Input: part model. Units: mm. Frame: model coordinates. A direction names the side the tool comes from. Round coordinates to 2 decimals unless told otherwise and drop trailing zeros. Order: outer loops, then holes, each group sorted by start corner. A loop starts at its lowest first (then second) coordinate and runs counter-clockwise, first axis right, second up. Notation, with made-up numbers: (39.5, 55.5) -> (62.5, 55.5) arc R4 ccw to (62.5, 61.5) -> close; hole circle Ø6 at (-14.5, 27.25). An arc over 180 degrees is marked (long way). Answer as CSV lines item,"result". Start each with the question number.
1) Section query A-A, the plane z = 44. Output: boundary loops of the cut face in (x, y), and give its area (3 significant figures).
2) Section query C-C, the plane y = 9. Output: boundary loops of the cut face in (x, z).
3) First-contact query: P1, Ø22, axis at y = 5, z = 32.5, coming from the -X side; P2, Ø16, axis at x = 28.5, y = 13, coming from the +Z side; P3, Ø5, axis at x = 25.5, z = 7.5, coming from the +Y side; P4, Ø6, axis at x = 46, y = 29.5, coming from the -Z side. Flat tips, straight axial feed; report the tip coordinate or a pass-through.
4) Line query: L1, parallel to X at y = 26.5, z = -34; L2, parallel to Y at x = 18, z = 19; L3, parallel to Y at x = 41, z = -26.5. Output: solid intervals per line, ascending.
5) Section query D-D, the plane x = 62.5. Output: boundary loops of the cut face in (y, z), and give its area (3 significant figures).
6) Access query for faces 1 (the face through (15, 20, -45)), 2 (the face through (20, 32, -30)), 3 (the face through (62.605, 9.86, 24.65)), 4 (the face through (50, 10, 35)), 5 (the face through (35, 23, -20)). Directions: +Z, -Z, +X, -X, +Y, -Y. A direction counts if a zero-diameter tool reaches every point of the face in a straight line with its end or side. Return the directions, or none.
7) Section query B-B, the plane y = 28.5. Output: boundary loops of the cut face in (x, z), and give its area (3 significant figures).
```python
from build123d import *

# Parameters (mm, degrees)
BOSS_EXTRUDE1_DEPTH = 20
SKETCH2_W           = 70
SKETCH2_H           = 30
BOSS_EXTRUDE2_DEPTH = 20
CUT_EXTRUDE1_REACH  = 96.868
SKETCH3_W           = 40
SKETCH3_H           = 10
CUT_EXTRUDE2_REACH  = 108.771
SKETCH4_W           = 30
SKETCH4_H           = 15


with BuildPart() as part:
    # Sketch1 → Boss-Extrude1 (new body)
    with BuildSketch(Plane(origin=(0, 0, 0), x_dir=(1, 0, 0), z_dir=(0, 1, 0))):
        Polygon((0, 0), (0, 50), (70, 50), (70, 0), (55, -50), (50, -50), (50, -20), (20, -20), (20, -50), (15, -50), align=None)
    extrude(amount=BOSS_EXTRUDE1_DEPTH)

    # Sketch2 → Boss-Extrude2 (add)
    with BuildSketch(Plane(origin=(0, 20, 0), x_dir=(1, 0, 0), z_dir=(0, 1, 0))):
        with Locations((35, 35)):
            Rectangle(SKETCH2_W, SKETCH2_H)
    extrude(amount=BOSS_EXTRUDE2_DEPTH)

    # Sketch3 → Cut-Extrude1 (cut, up to next)
    with BuildSketch(Plane(origin=(0, 40, 0), x_dir=(1, 0, 0), z_dir=(0, 1, 0)), mode=Mode.PRIVATE) as cut_extrude1_sk1:
        with Locations((35, 45)):
            Rectangle(SKETCH3_W, SKETCH3_H)
    cut_extrude1_tool1 = extrude(cut_extrude1_sk1.sketch, amount=-CUT_EXTRUDE1_REACH, mode=Mode.PRIVATE) & part.part
    add(cut_extrude1_tool1.solids().sort_by_distance((35, 40, -45))[0], mode=Mode.SUBTRACT)

    # Sketch4 → Cut-Extrude2 (cut, up to next)
    with BuildSketch(Plane.XY.offset(-20), mode=Mode.PRIVATE) as cut_extrude2_sk1:
        with Locations((35, 32.5)):
            Rectangle(SKETCH4_W, SKETCH4_H)
    cut_extrude2_tool1 = extrude(cut_extrude2_sk1.sketch, amount=-CUT_EXTRUDE2_REACH, mode=Mode.PRIVATE) & part.part
    add(cut_extrude2_tool1.solids().sort_by_distance((35, 32.5, -20))[0], mode=Mode.SUBTRACT)


solid = part.part
```
Findings:
1,outline,"(13.2, 0) -> (20, 0) -> (20, 20) -> (13.2, 20) -> close; (50, 0) -> (56.8, 0) -> (56.8, 20) -> (50, 20) -> close"
1,area,"272 mm^2"
2,outline,"(0, -50) -> (15, -50) -> (15, -40) -> (55, -40) -> (55, -50) -> (70, -50) -> (70, 0) -> (55, 50) -> (50, 50) -> (50, 20) -> (20, 20) -> (20, 50) -> (15, 50) -> (0, 0) -> close"
3,P1,"stops at x = 6.45"
3,P2,"stops at z = 20"
3,P3,"stops at y = 20"
3,P4,"passes through"
4,L1,"x = 0 to 20, 50 to 70"
4,L2,"y = 0 to 20"
4,L3,"y = 0 to 25"
5,outline,"(0, -50) -> (40, -50) -> (40, -20) -> (20, -20) -> (20, 25) -> (0, 25) -> close"
5,area,"2,100 mm^2"
6,face 1,"-Z, +Y, -Y"
6,face 2,"+Z, -Z, +Y"
6,face 3,"+Z, +X, +Y, -Y"
6,face 4,"+Z, +Y, -Y"
6,face 5,"+Z, +X, -X, +Y"
7,outline,"(0, -50) -> (15, -50) -> (15, -40) -> (20, -40) -> (20, -20) -> (0, -20) -> close; (50, -40) -> (55, -40) -> (55, -50) -> (70, -50) -> (70, -20) -> (50, -20) -> close"
7,area,"1,100 mm^2"
